Here's how the part is built. I have some questions about the finished solid (model axes, mm). Face numbers are marked on the shaded views. Round coordinates to 2 decimals unless told otherwise and drop trailing zeros. Order: outer loops, then holes, each group sorted by start corner. A loop starts at its lowest first (then second) coordinate and runs counter-clockwise, first axis right, second up. Notation, with made-up numbers: (75, 65.25) - (129, 65.25) arc R29 ccw to (129, 89.25) - close; hole circle Ø1 at (25.5, 61). An arc over 180 degrees is marked (long way). One line per item, written item: value.
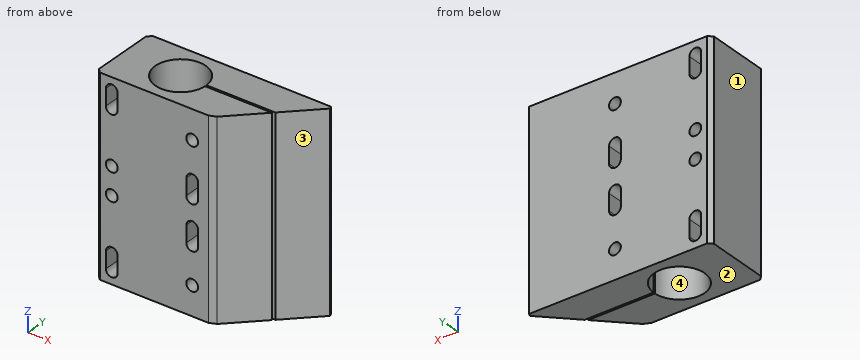
Autodesk Inventor part; units mm, degrees
ref_plane "YZ Plane" through (0, 0, 0) normal (1, 0, 0) x (0, 1, 0)
ref_plane "XZ Plane" through (0, 0, 0) normal (0, 1, 0) x (-1, 0, 0)
ref_plane "XY Plane" through (0, 0, 0) normal (0, 0, 1) x (1, 0, 0)
sketch "Sketch1" plane through (0, 0, 0) normal (0, 0, 1) x (1, 0, 0)
  line L0 (66, 18) -> (-30, 18) construction
  line L1 (-30, -18) -> (30, -18) construction
  line L2 (30, -18) -> (33.623, -14.377) construction
  line L3 (47.5, -0.5) -> (33.623, -14.377) construction
  line L4 (-30, 18) -> (-30, -18)
  line L5 (-30, -18) -> (30, -18)
  line L6 (30, -18) -> (47.5, -0.5)
  line L7 (47.5, -0.5) -> (12.9904, -0.5)
  line L8 (12.9904, 0.5) -> (48.5, 0.5)
  line L9 (48.5, 0.5) -> (66, 18)
  line L10 (66, 18) -> (-30, 18)
  arc A0 (12.9904, 0.5) -> (12.9904, -0.5) centre (0, 0) ccw
  line L11 (12.9904, 0.5) -> (12.9904, -0.5) construction
  point P0 (-30, 0)
  point P1 (18, 18)
  dimension "d2" = 36
  dimension "d4" = 60
  dimension "d5" = 135
  dimension "d7" = 13
  dimension "d10" = 1
  dimension "d12" = 30
extrude "Extrusion1" add sketch "Sketch1" along normal blind 100
sketch "Sketch2" plane through (-30, 18, 0) normal (0, 1, 0) x (1, 0, 0)
  line L0 (118, 0) -> (118, -100)
  line L1 (118, 0) -> (2, 0)
  line L2 (2, -100) -> (2, 0)
  line L3 (2, -100) -> (118, -100)
  line L4 (108.825, -15) -> (108.825, -6.5)
  arc A0 (114.925, -6.5) -> (108.825, -6.5) centre (111.875, -6.5) ccw
  line L5 (114.925, -6.5) -> (114.925, -15)
  arc A1 (108.825, -15) -> (114.925, -15) centre (111.875, -15) ccw
  line L6 (5.075, -15) -> (5.075, -6.5)
  arc A2 (11.175, -6.5) -> (5.075, -6.5) centre (8.125, -6.5) ccw
  line L7 (11.175, -6.5) -> (11.175, -15)
  arc A3 (5.075, -15) -> (11.175, -15) centre (8.125, -15) ccw
  circle A4 centre (49.625, -15) radius 3.05
  circle A5 centre (70.375, -15) radius 3.05
  circle A6 centre (70.375, -85) radius 3.05
  circle A7 centre (49.625, -85) radius 3.05
  line L8 (114.925, -85) -> (114.925, -93.5)
  arc A8 (108.825, -93.5) -> (114.925, -93.5) centre (111.875, -93.5) ccw
  line L9 (108.825, -93.5) -> (108.825, -85)
  arc A9 (114.925, -85) -> (108.825, -85) centre (111.875, -85) ccw
  circle A10 centre (111.875, -57.125) radius 3.05
  line L10 (67.325, -42.875) -> (67.325, -34.375)
  arc A11 (73.425, -34.375) -> (67.325, -34.375) centre (70.375, -34.375) ccw
  line L11 (73.425, -34.375) -> (73.425, -42.875)
  arc A12 (67.325, -42.875) -> (73.425, -42.875) centre (70.375, -42.875) ccw
  circle A13 centre (8.125, -42.875) radius 3.05
  circle A14 centre (111.875, -42.875) radius 3.05
  line L12 (46.575, -42.875) -> (46.575, -34.375)
  arc A15 (52.675, -34.375) -> (46.575, -34.375) centre (49.625, -34.375) ccw
  line L13 (52.675, -34.375) -> (52.675, -42.875)
  arc A16 (46.575, -42.875) -> (52.675, -42.875) centre (49.625, -42.875) ccw
  circle A17 centre (8.125, -57.125) radius 3.05
  line L14 (46.575, -65.625) -> (46.575, -57.125)
  arc A18 (52.675, -57.125) -> (46.575, -57.125) centre (49.625, -57.125) ccw
  line L15 (52.675, -57.125) -> (52.675, -65.625)
  arc A19 (46.575, -65.625) -> (52.675, -65.625) centre (49.625, -65.625) ccw
  line L16 (5.075, -93.5) -> (5.075, -85)
  arc A20 (11.175, -85) -> (5.075, -85) centre (8.125, -85) ccw
  line L17 (11.175, -85) -> (11.175, -93.5)
  arc A21 (5.075, -93.5) -> (11.175, -93.5) centre (8.125, -93.5) ccw
  line L18 (67.325, -65.625) -> (67.325, -57.125)
  arc A22 (73.425, -57.125) -> (67.325, -57.125) centre (70.375, -57.125) ccw
  line L19 (73.425, -57.125) -> (73.425, -65.625)
  arc A23 (67.325, -65.625) -> (73.425, -65.625) centre (70.375, -65.625) ccw
  point P0 (30, 0)
extrude "Extrusion2" cut sketch "Sketch2" against normal through all contours L6 A2 L7 A3 | A4 | A7 | A13 | L12 A15 L13 A16 | A17 | L14 A18 L15 A19 | L16 A20 L17 A21
chamfer "Chamfer1" distance 2 angle 45 4 edges at (-30, 18, 50) (-30, -18, 50) (66, 18, 50) (30, -18, 50)
properties part number "AXTSC" material "PC/ABS Plastic"
Q1. If we section it at C-C, the plane x = -20: Please give me the cut outline in (y, z), then the cut area to 3 significant figures.
Results list:
outline: (-18, 0) - (18, 0) - (18, 4.09) - (-18, 4.09) - close; (-18, 17.41) - (18, 17.41) - (18, 40.47) - (-18, 40.47) - close; (-18, 45.28) - (18, 45.28) - (18, 54.72) - (-18, 54.72) - close; (-18, 59.53) - (18, 59.53) - (18, 82.59) - (-18, 82.59) - close; (-18, 95.91) - (18, 95.91) - (18, 100) - (-18, 100) - close
area: 2,300 mm²
Q2. If we section it at B-B, the plane y = 6: Give the number of separate pieces and of enclosed holes in the cut face, then the cut area to 3 significant figures.
Results list:
separate pieces: 2
enclosed holes: 8
area: 5,650 mm²
Q3. We'd pull the mould along X, two halves only. Please class the marked faces 1, 2, 3 and 4: released by +X, released by -X, zero draft, split by the parting line, or undercut.
Results list:
face 1: released by -X
face 2: zero draft
face 3: released by +X
face 4: undercut
Q4. If we section it at D-D, the plane z = 72.5: Please give me the cut outline in (x, y), then the cut area to 3 significant figures.
Results list:
outline: (-30, -16) - (-28, -18) - (28, -18) - (31.41, -16.59) - (47.5, -0.5) - (12.99, -0.5) arc R13 cw (long way) to (12.99, 0.5) - (48.5, 0.5) - (64.59, 16.59) - (64, 18) - (-28, 18) - (-30, 16) - close
area: 2,240 mm²
Q5. If I drill on line 1 along Y through (x, z) = (17.5, 95); line 2 along X through (y, z) = (-7, 85) (3 decimals); line 3 along X through (y, z) = (12, 15) (3 decimals), over which ranges is the centre line in solid material (lowest first)?
Results list:
line 1: -18 to -0.5, 0.5 to 18
line 2: -30 to -24.925, -18.825 to -10.954, 10.954 to 16.575, 22.675 to 41
line 3: -30 to -24.925, -18.825 to -5, 5 to 16.575, 22.675 to 60
Q6. If we section it at A-A, the plane x = 37: Please give me the cut outline in (y, z).
Results list:
outline: (-11, 0) - (-0.5, 0) - (-0.5, 100) - (-11, 100) - close; (0.5, 0) - (18, 0) - (18, 100) - (0.5, 100) - close
Q7. Will these pins go through, and if not, where does the flat tip stop? pin 1 (2.5 mm diameter, centred on y = -7.5, z = 63, fed in from +X); pin 2 (9.5 mm diameter, centred on y = -9, z = 38.5, fed in from +X); pin 3 (7 mm diameter, centred on y = 6, z = 63, fed in from +X).
Results list:
pin 1: x = 41.75
pin 2: x = 43.75
pin 3: x = 57.5
